from build123d import *

# Parameters (mm, degrees)
SKETCH1_W           = 600
SKETCH1_H           = 60
BOSS_EXTRUDE1_DEPTH = 3
SKETCH3_W           = 600
SKETCH3_H           = 60
BOSS_EXTRUDE2_DEPTH = 3
SKETCH2_W           = 30
SKETCH2_H           = 3
SKETCH2_W_2         = 3
SKETCH2_H_2         = 30
CUT_EXTRUDE1_DEPTH  = 5
CUT_EXTRUDE2_DEPTH  = 5


with BuildPart() as part:
    # Sketch1 → Boss-Extrude1 (new body)
    with BuildSketch(Plane(origin=(0, 0, 0), x_dir=(1, 0, 0), z_dir=(0, 1, 0))):
        with Locations((300, 30)):
            Rectangle(SKETCH1_W, SKETCH1_H)
    extrude(amount=BOSS_EXTRUDE1_DEPTH)

    # Sketch3 → Boss-Extrude2 (add)
    with BuildSketch(Plane(origin=(0, 3, 0), x_dir=(1, 0, 0), z_dir=(0, 1, 0))):
        with Locations((300, -30)):
            Rectangle(SKETCH3_W, SKETCH3_H)
    extrude(amount=-BOSS_EXTRUDE2_DEPTH)

    # Sketch2 → Cut-Extrude1 (cut)
    with BuildSketch(Plane(origin=(0, 3, 0), x_dir=(1, 0, 0), z_dir=(0, 1, 0))):
        with Locations((0, 1.5)):
            Rectangle(SKETCH2_W, SKETCH2_H)
        with Locations((60, 1.5)):
            Rectangle(SKETCH2_W, SKETCH2_H)
        with Locations((120, 1.5)):
            Rectangle(SKETCH2_W, SKETCH2_H)
        with Locations((180, 1.5)):
            Rectangle(SKETCH2_W, SKETCH2_H)
        with Locations((240, 1.5)):
            Rectangle(SKETCH2_W, SKETCH2_H)
        with Locations((300, 1.5)):
            Rectangle(SKETCH2_W, SKETCH2_H)
        with Locations((360, 1.5)):
            Rectangle(SKETCH2_W, SKETCH2_H)
        with Locations((420, 1.5)):
            Rectangle(SKETCH2_W, SKETCH2_H)
        with Locations((480, 1.5)):
            Rectangle(SKETCH2_W, SKETCH2_H)
        with Locations((540, 1.5)):
            Rectangle(SKETCH2_W, SKETCH2_H)
        with Locations((540, 58.5)):
            Rectangle(SKETCH2_W, SKETCH2_H)
        with Locations((480, 58.5)):
            Rectangle(SKETCH2_W, SKETCH2_H)
        with Locations((420, 58.5)):
            Rectangle(SKETCH2_W, SKETCH2_H)
        with Locations((360, 58.5)):
            Rectangle(SKETCH2_W, SKETCH2_H)
        with Locations((300, 58.5)):
            Rectangle(SKETCH2_W, SKETCH2_H)
        with Locations((240, 58.5)):
            Rectangle(SKETCH2_W, SKETCH2_H)
        with Locations((180, 58.5)):
            Rectangle(SKETCH2_W, SKETCH2_H)
        with Locations((120, 58.5)):
            Rectangle(SKETCH2_W, SKETCH2_H)
        with Locations((60, 58.5)):
            Rectangle(SKETCH2_W, SKETCH2_H)
        with Locations((0, 58.5)):
            Rectangle(SKETCH2_W, SKETCH2_H)
        with Locations((1.5, 30)):
            Rectangle(SKETCH2_W_2, SKETCH2_H_2)
        with Locations((598.5, 30)):
            Rectangle(SKETCH2_W_2, SKETCH2_H_2)
        with Locations((600, 1.5)):
            Rectangle(SKETCH2_W, SKETCH2_H)
        with Locations((600, 58.5)):
            Rectangle(SKETCH2_W, SKETCH2_H)
    extrude(amount=-CUT_EXTRUDE1_DEPTH, mode=Mode.SUBTRACT)

    # Sketch4 → Cut-Extrude2 (cut)
    with BuildSketch(Plane(origin=(0, 3, 0), x_dir=(1, 0, 0), z_dir=(0, 1, 0))):
        with BuildLine():
            Line((80, -60), (520, -60))
            ThreePointArc((520, -60), (300, -20), (80, -60))
        make_face()
    extrude(amount=-CUT_EXTRUDE2_DEPTH, mode=Mode.SUBTRACT)


solid = part.part
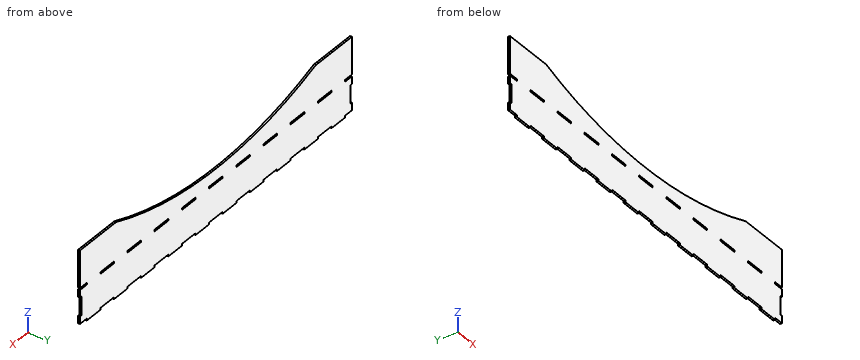
Work out the finished part from the listing and answer in its coordinate system (mm). Round coordinates to 2 decimals unless told otherwise and drop trailing zeros. Order: outer loops, then holes, each group sorted by start corner. A loop starts at its lowest first (then second) coordinate and runs counter-clockwise, first axis right, second up. Notation, with made-up numbers: M 81,47 L 97,47 A19 ccw 97,64 Z; hole C 67.5,59.5 d2. An arc over 180 degrees is marked long. Put each result on its own line as item: value. Start each with the question number.
Q1. Straight lines are drawn through the part: L1, parallel to Z at x = 302, y = 0.6; L2, parallel to Z at x = 553, y = 1.85; L3, parallel to X at y = 1.15, z = -31. For each, find the intervals that lie inside material, in ascending order. Write a range as [from, to].
Q2. Section C-C, the plane y = 1 is taken. Give the number of separate pieces and of enclosed holes in the cut face, and give its area (3 significant figures).
Q3. Section A-A, the plane z = 46 is taken. Write down the section's boundary in (x, y), and give its area (3 significant figures).
Q4. Flat-ended cylindrical pins translate along their axes: pin 1 (10 mm diameter, centred on x = 283, z = 8, fed in from -Y); pin 2 (0.9 mm diameter, centred on x = 240, y = 2, fed in from -Z); pin 3 (0.9 mm diameter, centred on y = 1, z = -1.5, fed in from +X); pin 4 (1.5 mm diameter, centred on y = 2, z = -59, fed in from -X). Find the tip coordinate at first contact, or state that the pin passes through.
Q5. Section B-B, the plane x = 121.5 is taken. Write down the section's boundary in (y, z).
Q6. Section D-D, the plane x = 336 is taken. Write down the section's boundary in (y, z), and give its area (3 significant figures).
Findings below:
1. L1: z = [-57, -3], [0, 20]
1. L2: z = [-57, -3], [0, 60]
1. L3: x = [3, 597]
2. separate pieces: 1
2. enclosed holes: 9
2. area: 58,200 mm^2
3. outline: M 0,0 L 121.61,0 L 121.61,3 L 0,3 Z; M 478.39,0 L 600,0 L 600,3 L 478.39,3 Z
3. area: 730 mm^2
4. pin 1: stops at y = 0
4. pin 2: stops at z = -57
4. pin 3: stops at x = 585
4. pin 4: stops at x = 15
5. outline: M 0,-57 L 3,-57 L 3,-3 L 0,-3 Z; M 0,0 L 3,0 L 3,46.03 L 0,46.03 Z
6. outline: M 0,-60 L 3,-60 L 3,21.04 L 0,21.04 Z
6. area: 243 mm^2
